Geometry: see drawing. Coordinates: mm, zero at the bounding-box minimum. Coordinates: 2 decimals unless noted, no trailing zeros. Order: outer loops, then holes, each group sorted by start corner. A loop starts at its lowest first (then second) coordinate and runs counter-clockwise, first axis right, second up.
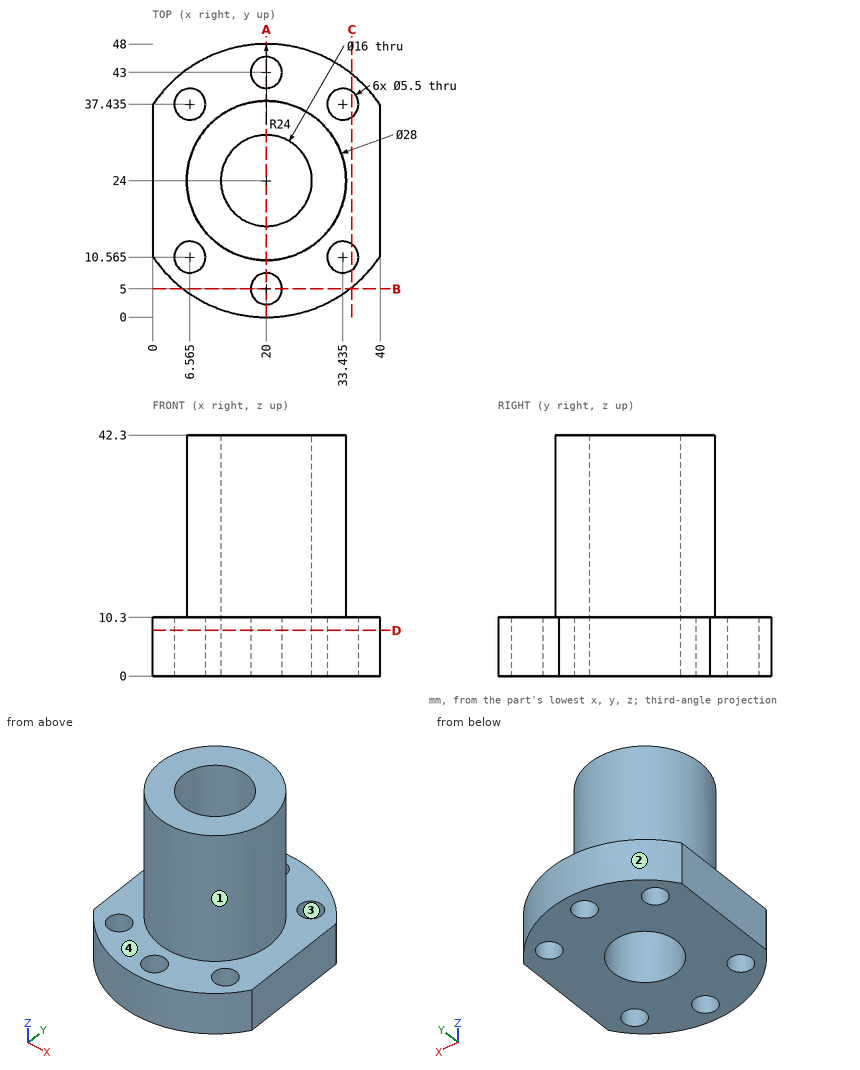
Q1. Section query B-B on y = 5. Output: boundary loops of the cut face in (x, z), plus the area to 3 significant figures.
Solutions:
outline: (5.34, 0) - (17.25, 0) - (17.25, 10.3) - (5.34, 10.3) - close; (22.75, 0) - (34.66, 0) - (34.66, 10.3) - (22.75, 10.3) - close
area: 245 mm2
Q2. Material intervals for line 1 along X through (y, z) = (38, 9.5); line 2 along Z through (x, y) = (3, 35); line 3 along X through (y, z) = (18, 3.5), sorted ascending.
Solutions:
line 1: x = 0.51 to 3.87, 9.26 to 30.74, 36.13 to 39.49
line 2: z = 0 to 10.3
line 3: x = 0 to 14.71, 25.29 to 40
Q3. Section query D-D on z = 8. Give the number of separate pieces and of enclosed holes in the cut face, plus the area to 3 significant figures.
Solutions:
separate pieces: 1
enclosed holes: 7
area: 1,320 mm2
Q4. Pin query (flat end, axial travel): P1, Ø4, axis at x = 14, z = 35.5, coming from the -Y side; P2, Ø5, axis at y = 40, z = 7.5, coming from the +X side; P3, Ø3, axis at x = 14.5, z = 18.5, coming from the +Y side. Return the tip coordinate at first contact, or that it passes through.
Solutions:
P1: stops at y = 10.58
P2: stops at x = 39.84
P3: stops at y = 37.42
Q5. Pull-direction query (Y, two-part tool) for the marked faces 1, 2, 3 and 4; classes: pulls with the +Y half, pulls with the -Y half, needs draft (parallel to the pull), parting line crosses it, or undercut.
Solutions:
face 1: parting line crosses it
face 2: pulls with the +Y half
face 3: undercut
face 4: needs draft
Q6. Section query A-A on x = 20. Output: boundary loops of the cut face in (y, z).
Solutions:
outline: (0, 0) - (2.25, 0) - (2.25, 10.3) - (0, 10.3) - close; (7.75, 0) - (16, 0) - (16, 42.3) - (10, 42.3) - (10, 10.3) - (7.75, 10.3) - close; (32, 0) - (40.25, 0) - (40.25, 10.3) - (38, 10.3) - (38, 42.3) - (32, 42.3) - close; (45.75, 0) - (48, 0) - (48, 10.3) - (45.75, 10.3) - close
Q7. Section query C-C on x = 35. Output: boundary loops of the cut face in (y, z) (3 decimals).
Solutions:
outline: (5.265, 0) - (8.304, 0) - (8.304, 10.3) - (5.265, 10.3) - close; (12.826, 0) - (35.174, 0) - (35.174, 10.3) - (12.826, 10.3) - close; (39.696, 0) - (42.735, 0) - (42.735, 10.3) - (39.696, 10.3) - close
